For this review, use the dimensioned drawing (mm, ordinates from the lowest corner) and the shaded views. A direction names the side the tool comes from. Give positions to 0.01 mm unless a question says otherwise; leave off trailing zeros. Order: outer loops, then holes, each group sorted by start corner. A loop starts at its lowest first (then second) coordinate and runs counter-clockwise, first axis right, second up. Notation, with made-up numbers: (32.5, 78) - (48.5, 78) arc R37 ccw to (48.5, 114) - close; hole circle Ø9 at (37, 31). An arc over 180 degrees is marked (long way). Answer as CSV lines item,"result". Start each with the question number.
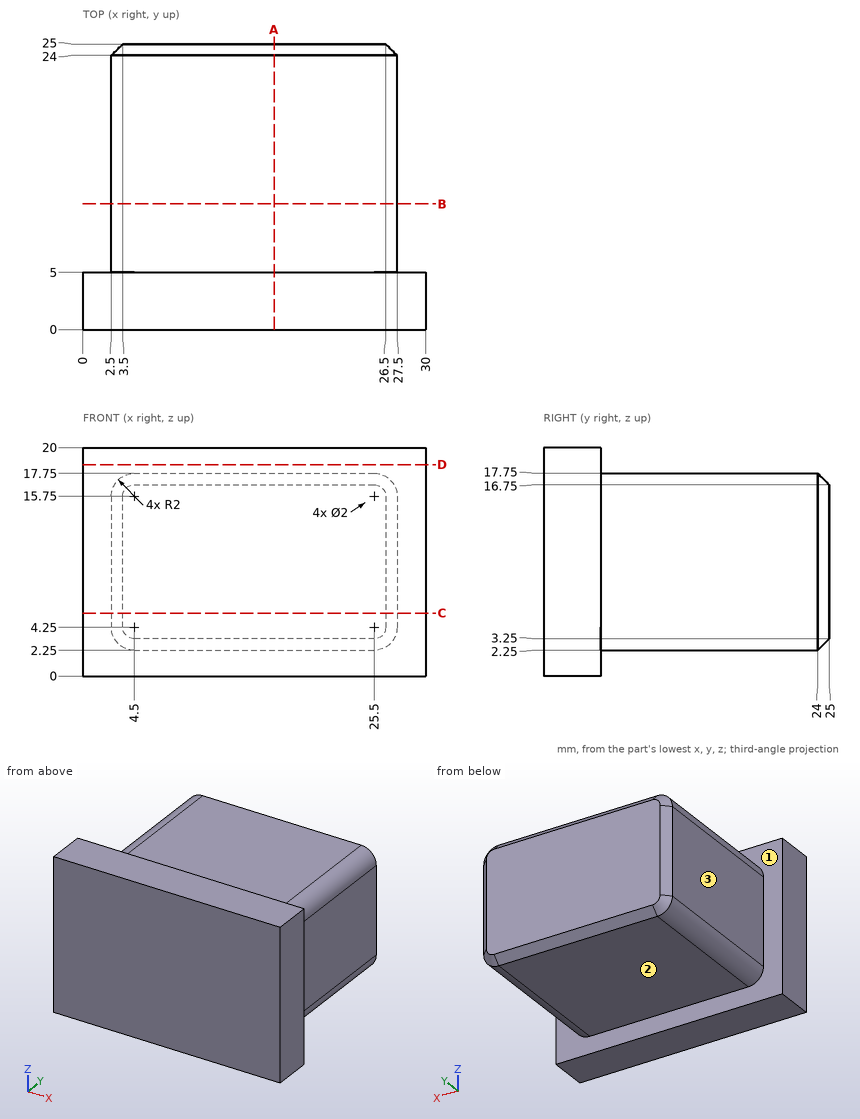
Item 1: Take a section at C-C on z = 5.5. Write out the cut boundary in (x, y), and give its area (3 significant figures).
Item 2: For line 1 along Y through (x, z) = (28.75, 6); line 2 along Z through (x, y) = (19.25, 22.75); line 3 along X through (y, z) = (23.75, 11.5), list the stretches that pass through material, from the lowest coordinate up.
Item 3: Take a section at A-A on x = 16.75. Write out the cut boundary in (y, z).
Item 4: Clearance check with flat-ended pins moving along their axes: pin 1 (1.5 mm diameter, centred on x = 15.5, y = 6.5, fed in from +Z); pin 2 (3.5 mm diameter, centred on y = 14.5, z = 11.5, fed in from +X); pin 3 (9.5 mm diameter, centred on x = 12, y = 11.5, fed in from -Z). State where each tip first meets the part, or that it passes through.
Item 5: Take a section at B-B on y = 11. Write out the cut boundary in (x, z).
Item 6: Take a section at D-D on z = 18.5. Write out the cut boundary in (x, y).
Item 7: Machinability: for the marked faces 1, 2 and 3, which of the approach directions +Z, -Z, +X, -X, +Y, -Y give a long, thin tool a straight path to every point of the face, cutting with its end or side? Answer none if there is none.
Data:
1,outline,"(0, 0) - (30, 0) - (30, 5) - (27.5, 5) - (27.5, 24) - (26.5, 25) - (3.5, 25) - (2.5, 24) - (2.5, 5) - (0, 5) - close"
1,area,"649 mm^2"
2,line 1,"y = 0 to 5"
2,line 2,"z = 2.25 to 17.75"
2,line 3,"x = 2.5 to 27.5"
3,outline,"(0, 0) - (5, 0) - (5, 2.25) - (24, 2.25) - (25, 3.25) - (25, 16.75) - (24, 17.75) - (5, 17.75) - (5, 20) - (0, 20) - close"
4,pin 1,"stops at z = 17.75"
4,pin 2,"stops at x = 27.5"
4,pin 3,"stops at z = 2.25"
5,outline,"(2.5, 4.25) arc R2 ccw to (4.5, 2.25) - (25.5, 2.25) arc R2 ccw to (27.5, 4.25) - (27.5, 15.75) arc R2 ccw to (25.5, 17.75) - (4.5, 17.75) arc R2 ccw to (2.5, 15.75) - close"
6,outline,"(0, 0) - (30, 0) - (30, 5) - (0, 5) - close"
7,face 1,"+Y"
7,face 2,"-Z, +X, -X, +Y"
7,face 3,"+Z, -Z, -X, +Y"
